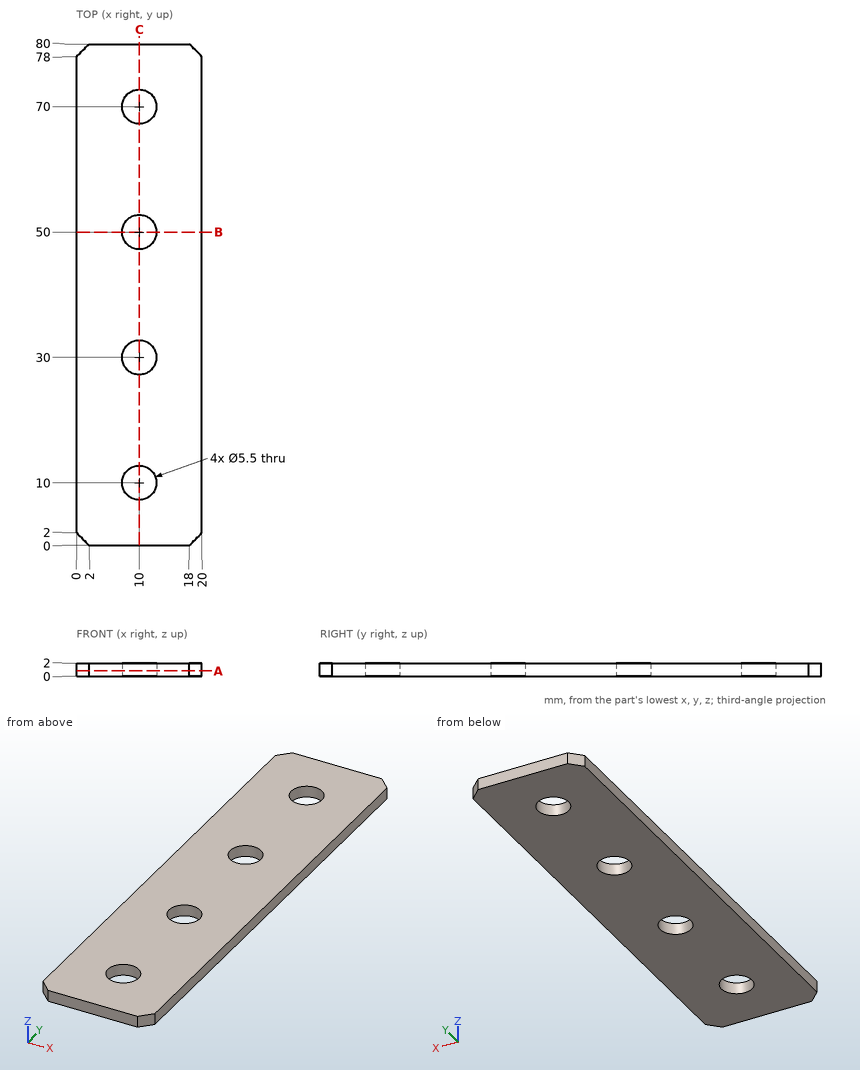
Geometry check sheet. Reference: drawing and pictorial views, mm from the part's lowest x, y, z. Coordinates: 2 decimals unless noted, no trailing zeros. Order: outer loops, then holes, each group sorted by start corner. A loop starts at its lowest first (then second) coordinate and runs counter-clockwise, first axis right, second up.
1. Sectioned sample at A-A, the plane z = 0.8. Record the cut outline in (x, y), and give its area (3 significant figures).
Results found:
outline: (0, 2) - (2, 0) - (18, 0) - (20, 2) - (20, 78) - (18, 80) - (2, 80) - (0, 78) - close; hole circle Ø5.5 at (10, 10); hole circle Ø5.5 at (10, 30); hole circle Ø5.5 at (10, 50); hole circle Ø5.5 at (10, 70)
area: 1,500 mm2
2. Go/stop test with a flat-tipped pin: pin 1 Ø4.5 at (x, y) = (10, 50) entering from -Z. Record where the tip stops, or that it passes through.
Results found:
pin 1: passes through
3. Sectioned sample at B-B, the plane y = 50. Record the cut outline in (x, z), and give its area (3 significant figures).
Results found:
outline: (0, 0) - (7.25, 0) - (7.25, 2) - (0, 2) - close; (12.75, 0) - (20, 0) - (20, 2) - (12.75, 2) - close
area: 29.0 mm2
4. Scan lines: line 1 (Y direction, x = 10, z = 1.25); line 2 (Y direction, x = 8.75, z = 0.2); line 3 (X direction, y = 51.5, z = 0.6). Record each from-to range of solid material in increasing order.
Results found:
line 1: y = 0 to 7.25, 12.75 to 27.25, 32.75 to 47.25, 52.75 to 67.25, 72.75 to 80
line 2: y = 0 to 7.55, 12.45 to 27.55, 32.45 to 47.55, 52.45 to 67.55, 72.45 to 80
line 3: x = 0 to 7.7, 12.3 to 20
5. Sectioned sample at C-C, the plane x = 10. Record the cut outline in (y, z).
Results found:
outline: (0, 0) - (7.25, 0) - (7.25, 2) - (0, 2) - close; (12.75, 0) - (27.25, 0) - (27.25, 2) - (12.75, 2) - close; (32.75, 0) - (47.25, 0) - (47.25, 2) - (32.75, 2) - close; (52.75, 0) - (67.25, 0) - (67.25, 2) - (52.75, 2) - close; (72.75, 0) - (80, 0) - (80, 2) - (72.75, 2) - close
